Could you check a few things on this model? Use its own coordinates, in mm. Coordinates: 2 decimals unless noted, no trailing zeros. Order: outer loops, then holes, each group sorted by start corner. A loop starts at its lowest first (then second) coordinate and runs counter-clockwise, first axis right, second up. Notation, with made-up numbers: (-26.5, 89) -> (6.5, 89) arc R28 ccw to (6.5, 108) -> close; hole circle Ø1 at (6.5, -23). An arc over 180 degrees is marked (long way). Use a Markdown table: item, result. Add a question column.
1) If we section it at D-D (y = -1.3): Give the number of separate pieces and of enclosed holes in the cut face, plus the area to 3 significant figures.
2) Will these pins go through, and if not, where does the flat tip stop? pin 1 Ø3 at (x, z) = (9, -33.25) entering from -Y; pin 2 Ø1.2 at (x, y) = (-2.5, 1) entering from -Z; pin 3 Ø2 at (y, z) = (-0.5, -52.5) entering from +X; pin 4 Ø1.2 at (y, z) = (0, -11.5) entering from +X.
3) If we section it at A-A (z = 76): Write out the boundary of the cut face in (x, y).
4) Thinking about a two-plate mould opening in X: for faces 1 (the flat face through (35.34, -0.03, 49.27)), 2 (the flat face through (-1, 2, 18)), which applies, +X half, -X half, draft (parallel to the pull), parting line (faces both ways), or undercut?
5) If I drill on L1, parallel to X at y = 1.75, z = 43.5; L2, parallel to Z at x = 33, y = -0.05; L3, parallel to X at y = 1.65, z = 46, over which ranges is the centre line in solid material (lowest first)? Write a range as [from, to].
6) If we section it at C-C (x = -48): Write out the boundary of the cut face in (y, z), plus the area to 3 significant figures.
7) If we section it at B-B (z = 3): Write out the boundary of the cut face in (x, y), plus the area to 3 significant figures.
```python
from build123d import *

# Parameters (mm, degrees)
SKETCH1_R           = 85
SKETCH1_R_2         = 2.05
SKETCH1_R_3         = 1.55
SKETCH1_W           = 50
SKETCH1_H           = 35
BOSS_EXTRUDE1_DEPTH = 2
SKETCH2_R           = 1.15
SKETCH2_R_2         = 1.150012437
CUT_EXTRUDE1_DEPTH  = 5
CUT_EXTRUDE2_START  = -4
CUT_EXTRUDE2_DEPTH  = 4
CUT_EXTRUDE3_REACH  = 6
SKETCH4_W           = 8
SKETCH4_H           = 5.5


with BuildPart() as part:
    # Sketch1 → Boss-Extrude1 (new body, symmetric)
    with BuildSketch(Plane(origin=(0, 0, 0), x_dir=(1, 0, 0), z_dir=(0, 1, 0))):
        Circle(SKETCH1_R)
        with Locations((65.817930688, 38)):
            Circle(SKETCH1_R_2, mode=Mode.SUBTRACT)
        with Locations((0, -76)):
            Circle(SKETCH1_R_2, mode=Mode.SUBTRACT)
        with Locations((-65.817930688, 38)):
            Circle(SKETCH1_R_2, mode=Mode.SUBTRACT)
        with Locations((43.301270189, 25)):
            Circle(SKETCH1_R_3, mode=Mode.SUBTRACT)
        with Locations((0, -50)):
            Circle(SKETCH1_R_3, mode=Mode.SUBTRACT)
        with Locations((-43.301270189, 25)):
            Circle(SKETCH1_R_3, mode=Mode.SUBTRACT)
        Polygon((75.286841774, -14.599364905), (50.286841774, -57.900635095), (19.975952642, -40.400635095), (44.975952642, 2.900635095), align=None, mode=Mode.SUBTRACT)
        with Locations((0, 55)):
            Rectangle(SKETCH1_W, SKETCH1_H, mode=Mode.SUBTRACT)
        Polygon((-50.286841774, -57.900635095), (-75.286841774, -14.599364905), (-44.975952642, 2.900635095), (-19.975952642, -40.400635095), align=None, mode=Mode.SUBTRACT)
        with BuildLine():
            Line((17.923393759, 0.044228634), (8.923393759, -15.544228634))
            Line((8.923393759, -15.544228634), (0.263139721, -10.544228634))
            Line((0.263139721, -10.544228634), (1.201188009, -8.91948134))
            ThreePointArc((1.201188009, -8.91948134), (0, -9), (-1.201188009, -8.91948134))
            Line((-1.201188009, -8.91948134), (-0.263139721, -10.544228634))
            Line((-0.263139721, -10.544228634), (-8.923393759, -15.544228634))
            Line((-8.923393759, -15.544228634), (-17.923393759, 0.044228634))
            Line((-17.923393759, 0.044228634), (-9.263139721, 5.044228634))
            Line((-9.263139721, 5.044228634), (-8.325091433, 3.41948134))
            ThreePointArc((-8.325091433, 3.41948134), (-7.794228634, 4.5), (-7.123903424, 5.5))
            Line((-7.123903424, 5.5), (-9, 5.5))
            Line((-9, 5.5), (-9, 15.5))
            Line((-9, 15.5), (9, 15.5))
            Line((9, 15.5), (9, 5.5))
            Line((9, 5.5), (7.123903424, 5.5))
            ThreePointArc((7.123903424, 5.5), (7.794228634, 4.5), (8.325091433, 3.41948134))
            Line((8.325091433, 3.41948134), (9.263139721, 5.044228634))
            Line((9.263139721, 5.044228634), (17.923393759, 0.044228634))
        make_face(mode=Mode.SUBTRACT)
    extrude(amount=BOSS_EXTRUDE1_DEPTH, both=True)

    # Sketch2 → Cut-Extrude1 (cut, through all)
    with BuildSketch(Plane(origin=(0, 2, 0), x_dir=(1, 0, 0), z_dir=(0, 1, 0))):
        with Locations((-9, 33.25)):
            Circle(SKETCH2_R)
        with Locations((9, 33.25)):
            Circle(SKETCH2_R)
        with Locations((-33.295344676, -8.830771366)):
            Circle(SKETCH2_R)
        with Locations((-24.295344676, -24.419228634)):
            Circle(SKETCH2_R)
        with Locations((24.295355446, -24.419234852)):
            Circle(SKETCH2_R_2)
        with Locations((33.295344676, -8.830771366)):
            Circle(SKETCH2_R)
    extrude(amount=-CUT_EXTRUDE1_DEPTH, mode=Mode.SUBTRACT)

    # Sketch3 → Cut-Extrude2 (cut)
    with BuildSketch(Plane(origin=(0, 2, 0), x_dir=(1, 0, 0), z_dir=(0, 1, 0)).offset(CUT_EXTRUDE2_START)):
        Polygon((9, 7.5), (-9, 7.5), (-10.995190528, 4.044228634), (-1.995190528, -11.544228634), (1.995190528, -11.544228634), (10.995190528, 4.044228634), align=None)
    extrude(amount=CUT_EXTRUDE2_DEPTH, mode=Mode.SUBTRACT)

    # Sketch4 → Cut-Extrude3 (cut, up to next)
    with BuildSketch(Plane(origin=(0, 2, 0), x_dir=(1, 0, 0), z_dir=(0, 1, 0)), mode=Mode.PRIVATE) as cut_extrude3_sk1:
        Polygon((64.786841774, -32.785898385), (69.549981495, -35.535898385), (65.549981495, -42.464101615), (60.786841774, -39.714101615), align=None)
    cut_extrude3_tool1 = extrude(cut_extrude3_sk1.sketch, amount=-CUT_EXTRUDE3_REACH, mode=Mode.PRIVATE) & part.part
    add(cut_extrude3_tool1.solids().sort_by_distance((65.168412, 2, 37.625))[0], mode=Mode.SUBTRACT)
    # Sketch4 → Cut-Extrude3 (cut, up to next)
    with BuildSketch(Plane(origin=(0, 2, 0), x_dir=(1, 0, 0), z_dir=(0, 1, 0)), mode=Mode.PRIVATE) as cut_extrude3_sk2:
        Polygon((-60.786841774, -39.714101615), (-64.786841774, -32.785898385), (-69.549981495, -35.535898385), (-65.549981495, -42.464101615), align=None)
    cut_extrude3_tool2 = extrude(cut_extrude3_sk2.sketch, amount=-CUT_EXTRUDE3_REACH, mode=Mode.PRIVATE) & part.part
    add(cut_extrude3_tool2.solids().sort_by_distance((-65.168412, 2, 37.625))[0], mode=Mode.SUBTRACT)
    # Sketch4 → Cut-Extrude3 (cut, up to next)
    with BuildSketch(Plane(origin=(0, 2, 0), x_dir=(1, 0, 0), z_dir=(0, 1, 0)), mode=Mode.PRIVATE) as cut_extrude3_sk3:
        with Locations((0, 75.25)):
            Rectangle(SKETCH4_W, SKETCH4_H)
    cut_extrude3_tool3 = extrude(cut_extrude3_sk3.sketch, amount=-CUT_EXTRUDE3_REACH, mode=Mode.PRIVATE) & part.part
    add(cut_extrude3_tool3.solids().sort_by_distance((0, 2, -75.25))[0], mode=Mode.SUBTRACT)


solid = part.part
```
Answer sheet:
| question | item | result |
|---|---|---|
| 1 | separate pieces | 1 |
| 1 | enclosed holes | 16 |
| 1 | area | 16,500 mm2 |
| 2 | pin 1 | y = -2 |
| 2 | pin 2 | z = -84.98 |
| 2 | pin 3 | x = 67.62 |
| 2 | pin 4 | x = 84.3 |
| 3 | outline | (-38.07, -2) -> (-2.05, -2) -> (-2.05, 2) -> (-38.07, 2) -> close; (2.05, -2) -> (38.07, -2) -> (38.07, 2) -> (2.05, 2) -> close |
| 4 | face 1 | undercut |
| 4 | face 2 | draft |
| 5 | L1 | [-73.03, -58.6], [-25.34, 25.34], [58.6, 73.03] |
| 5 | L2 | [-78.33, 7.72], [9.94, 17.84], [47.92, 78.33] |
| 5 | L3 | [-71.48, -57.16], [-29.67, 29.67], [57.16, 71.48] |
| 6 | outline | (-2, -70.15) -> (2, -70.15) -> (2, -1.15) -> (-2, -1.15) -> close; (-2, 56.58) -> (2, 56.58) -> (2, 70.15) -> (-2, 70.15) -> close |
| 6 | area | 330 mm2 |
| 7 | outline | (-84.95, -2) -> (-55.2, -2) -> (-55.2, 2) -> (-84.95, 2) -> close; (-41.57, -2) -> (-16.17, -2) -> (-16.17, 2) -> (-41.57, 2) -> close; (16.17, -2) -> (41.57, -2) -> (41.57, 2) -> (16.17, 2) -> close; (55.2, -2) -> (84.95, -2) -> (84.95, 2) -> (55.2, 2) -> close |
| 7 | area | 441 mm2 |
